from build123d import *

# Parameters (mm, degrees)
SKIZZE1_R                       = 59.5
AUFSATZ_LINEAR_AUSTRAGEN1_DEPTH = 2
SKIZZE2_R                       = 1.6
SKIZZE2_W                       = 75
SKIZZE2_H                       = 2.2
SKIZZE2_W_2                     = 2.2
SKIZZE2_H_2                     = 30.5
SCHNITT_LINEAR_AUSTRAGEN1_DEPTH = 2
SKIZZE3_R                       = 1.5
SKIZZE3_W                       = 75
SKIZZE3_H                       = 13.30476215
SKIZZE3_W_2                     = 5.981311675
SKIZZE3_H_2                     = 52
SCHNITT_LINEAR_AUSTRAGEN2_DEPTH = 2


with BuildPart() as part:
    # Skizze1 → Aufsatz-Linear austragen1 (new body)
    with BuildSketch(Plane.XY):
        Circle(SKIZZE1_R)
    extrude(amount=AUFSATZ_LINEAR_AUSTRAGEN1_DEPTH)

    # Skizze2 → Schnitt-Linear austragen1 (cut)
    with BuildSketch(Plane.XY.offset(2)):
        with Locations((37.5, -37.5)):
            Circle(SKIZZE2_R)
        with Locations((-37.5, -37.5)):
            Circle(SKIZZE2_R)
        with Locations((-37.5, 37.5)):
            Circle(SKIZZE2_R)
        with Locations((37.5, 37.5)):
            Circle(SKIZZE2_R)
        with Locations((-5.697175449, 27.6)):
            Rectangle(SKIZZE2_W, SKIZZE2_H)
        with Locations((-5.697175449, -27.6)):
            Rectangle(SKIZZE2_W, SKIZZE2_H)
        with Locations((-47.758902381, 0)):
            Rectangle(SKIZZE2_W_2, SKIZZE2_H_2)
    extrude(amount=-SCHNITT_LINEAR_AUSTRAGEN1_DEPTH, mode=Mode.SUBTRACT)

    # Skizze3 → Schnitt-Linear austragen2 (cut)
    with BuildSketch(Plane.XY.offset(2)):
        with Locations((-13, -42.7)):
            Circle(SKIZZE3_R)
        with Locations((13, -42.7)):
            Circle(SKIZZE3_R)
        with Locations((-13, 42.7)):
            Circle(SKIZZE3_R)
        with Locations((13, 42.7)):
            Circle(SKIZZE3_R)
        with Locations((0, 52.847618925)):
            Rectangle(SKIZZE3_W, SKIZZE3_H)
        with Locations((0, -52.847618925)):
            Rectangle(SKIZZE3_W, SKIZZE3_H)
        with Locations((-56.509344163, 0)):
            Rectangle(SKIZZE3_W_2, SKIZZE3_H_2)
    extrude(amount=-SCHNITT_LINEAR_AUSTRAGEN2_DEPTH, mode=Mode.SUBTRACT)


solid = part.part
Verification items for the finished model (mm, model axes). Give positions to 0.01 mm unless a question says otherwise; leave off trailing zeros. Write each loop counter-clockwise with the first axis right and the second up, starting at its lowest first coordinate (ties: lowest second). Pieces come first, ordered by that corner, then holes. Notation, with made-up numbers: M 10.5,-32.5 L 67.5,-32.5 A11 ccw 67.5,-12.5 Z; hole C 29,11 d5. An arc over 180 degrees is marked long. Write item = value, one per line.
(1) Material ranges on line 1 (Y direction, x = -13, z = 1.25); line 2 (Y direction, x = -37.5, z = 0.7); line 3 (Y direction, x = 37.5, z = 0.7), recorded low to high.
Found:
line_1 = -46.2 to -44.2, -41.2 to -28.7, -26.5 to 26.5, 28.7 to 41.2, 44.2 to 46.2
line_2 = -46.2 to -39.1, -35.9 to -28.7, -26.5 to 26.5, 28.7 to 35.9, 39.1 to 46.2
line_3 = -46.2 to -39.1, -35.9 to 35.9, 39.1 to 46.2
(2) Sectioned sample at D-D (y = -42.7). Record the cut outline in (x, z), then the cut area to 3 significant figures.
Found:
outline = M -41.44,0 L -14.5,0 L -14.5,2 L -41.44,2 Z; M -11.5,0 L 11.5,0 L 11.5,2 L -11.5,2 Z; M 14.5,0 L 41.44,0 L 41.44,2 L 14.5,2 Z
area = 154 mm2
(3) Sectioned sample at C-C (y = -13.5). Record the cut outline in (x, z).
Found:
outline = M -53.52,0 L -48.86,0 L -48.86,2 L -53.52,2 Z; M -46.66,0 L 57.95,0 L 57.95,2 L -46.66,2 Z
(4) Sectioned sample at A-A (z = 0.5). Give the number of separate pieces and of enclosed holes in the cut face, then the cut area to 3 significant figures.
Found:
separate_pieces = 1
enclosed_holes = 11
area = 9,090 mm2
(5) Sectioned sample at B-B (x = 7.5). Record the cut outline in (y, z), then the cut area to 3 significant figures.
Found:
outline = M -46.2,0 L -28.7,0 L -28.7,2 L -46.2,2 Z; M -26.5,0 L 26.5,0 L 26.5,2 L -26.5,2 Z; M 28.7,0 L 46.2,0 L 46.2,2 L 28.7,2 Z
area = 176 mm2
(6) Draft check along Y on faces 1 (the face through (59.495, -0.74, 0.986)), 2 (the face through (38.24, 36.08, 1.01)), 3 (the face through (38.24, -38.92, 1.01)), 4 (the face through (-46.73, -36.83, 0.99)). Enter one of: released by +Y, released by -Y, zero draft, split by the parting line, or undercut.
Found:
face_1 = split by the parting line
face_2 = undercut
face_3 = undercut
face_4 = released by -Y
(7) Go/stop test with flat-tipped pins: pin 1 Ø8 at (x, y) = (-35, -10) entering from -Z; pin 2 Ø0.6 at (x, z) = (-48, 1) entering from -Y; pin 3 Ø1 at (y, z) = (-27.5, 1.5) entering from +X; pin 4 Ø2.5 at (x, y) = (-13, -42.7) entering from +Z. Record where each tip stops, or that it passes through.
Found:
pin_1 = 0
pin_2 = -35.57
pin_3 = 53.02
pin_4 = through
